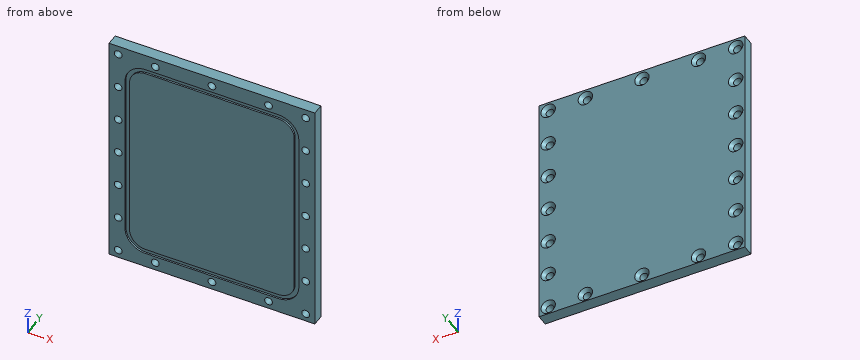
```python
from build123d import *

# Parameters (mm, degrees)
SKETCH1_W                                           = 90
SKETCH1_H                                           = 105
EXTRUDE1_DEPTH                                      = 5
CSK_FOR_M3_COUNTERSUNK_FLAT_HEAD_SCREW1_D           = 3.4
CSK_FOR_M3_COUNTERSUNK_FLAT_HEAD_SCREW1_CSINK_D     = 6.3
CSK_FOR_M3_COUNTERSUNK_FLAT_HEAD_SCREW1_CSINK_ANGLE = 90
EXTRUDE2_START                                      = -5
EXTRUDE2_DEPTH                                      = 0.75


with BuildPart() as part:
    # Sketch1 → Extrude1 (new body)
    with BuildSketch(Plane(origin=(0, 0, 0), x_dir=(1, 0, 0), z_dir=(0, 1, 0))):
        with Locations((45, 52.5)):
            Rectangle(SKETCH1_W, SKETCH1_H)
    extrude(amount=EXTRUDE1_DEPTH)

    # CSK for M3 Countersunk Flat Head Screw1 (through all)
    with Locations(Plane(origin=(4, 5, -4), x_dir=(0, 0, 1), z_dir=(0, 1, 0))):
        with Locations((0, 0), (-16.25, 0), (-32.5, 0), (-48.75, 0), (-65, 0), (-81.25, 0), (-97.5, 0), (-97.5, 16.25), (-97.5, 41), (-97.5, 65.75), (-97.5, 82), (-81.25, 82), (-65, 82), (-48.75, 82), (-32.5, 82), (-16.25, 82), (0, 82), (0, 65.75), (0, 41), (0, 16.25)):
            CounterSinkHole(CSK_FOR_M3_COUNTERSUNK_FLAT_HEAD_SCREW1_D / 2, CSK_FOR_M3_COUNTERSUNK_FLAT_HEAD_SCREW1_CSINK_D / 2, counter_sink_angle=CSK_FOR_M3_COUNTERSUNK_FLAT_HEAD_SCREW1_CSINK_ANGLE)

    # Sketch2 → Extrude2 (cut)
    with BuildSketch(Plane(origin=(0, 5, 0), x_dir=(1, 0, 0), z_dir=(0, 1, 0)).offset(EXTRUDE2_START)):
        with BuildLine():
            Line((16, 7), (74, 7))
            ThreePointArc((74, 7), (80.363961031, 9.636038969), (83, 16))
            Line((83, 16), (83, 89.5))
            ThreePointArc((83, 89.5), (80.363961031, 95.863961031), (74, 98.5))
            Line((74, 98.5), (16, 98.5))
            ThreePointArc((16, 98.5), (9.636038969, 95.863961031), (7, 89.5))
            Line((7, 89.5), (7, 16))
            ThreePointArc((7, 16), (9.636038969, 9.636038969), (16, 7))
        make_face()
        with BuildLine():
            Line((9, 89.5), (9, 16))
            ThreePointArc((9, 16), (11.050252532, 11.050252532), (16, 9))
            Line((16, 9), (74, 9))
            ThreePointArc((74, 9), (78.949747468, 11.050252532), (81, 16))
            Line((81, 16), (81, 89.5))
            ThreePointArc((81, 89.5), (78.949747468, 94.449747468), (74, 96.5))
            Line((74, 96.5), (16, 96.5))
            ThreePointArc((16, 96.5), (11.050252532, 94.449747468), (9, 89.5))
        make_face(mode=Mode.SUBTRACT)
    extrude(amount=EXTRUDE2_DEPTH, mode=Mode.SUBTRACT)


solid = part.part
```
Build history of the part. All positions in model axes, mm. Round coordinates to 2 decimals unless told otherwise and drop trailing zeros. Order: outer loops, then holes, each group sorted by start corner. A loop starts at its lowest first (then second) coordinate and runs counter-clockwise, first axis right, second up. Notation, with made-up numbers: (27.5, 52) -> (61.5, 52) arc R37 ccw to (61.5, 90) -> close; hole circle Ø8 at (35, -12). An arc over 180 degrees is marked (long way). Answer in a Markdown table with one row per item.
1) Band-saw the part on D-D on z = -69. Give the cut face in (x, y).
Values:
| item | result |
|---|---|
| outline | (0, 0) -> (2.3, 0) -> (2.3, 3.55) -> (0.85, 5) -> (0, 5) -> close; (5.7, 0) -> (7, 0) -> (7, 0.75) -> (9, 0.75) -> (9, 0) -> (81, 0) -> (81, 0.75) -> (83, 0.75) -> (83, 0) -> (84.3, 0) -> (84.3, 3.55) -> (82.85, 5) -> (7.15, 5) -> (5.7, 3.55) -> close; (87.7, 0) -> (90, 0) -> (90, 5) -> (89.15, 5) -> (87.7, 3.55) -> close |
2) Pin check, flat tips, straight feed: P1, Ø2, axis at x = 86, z = -20.25, coming from the -Y side; P2, Ø4, axis at x = 86, z = -4, coming from the +Y side; P3, Ø5.5, axis at x = 86, z = -52.75, coming from the +Y side. Stop position of each tip, or through.
Values:
| item | result |
|---|---|
| P1 | through |
| P2 | y = 3.85 |
| P3 | y = 4.6 |
3) Band-saw the part on B-B on x = 20.25. Give the cut face in (y, z), and give its area (3 significant figures).
Values:
| item | result |
|---|---|
| outline | (0, -105) -> (5, -105) -> (5, -104.65) -> (3.55, -103.2) -> (0, -103.2) -> close; (0, -99.8) -> (3.55, -99.8) -> (5, -98.35) -> (5, -7.15) -> (3.55, -5.7) -> (0, -5.7) -> (0, -7) -> (0.75, -7) -> (0.75, -9) -> (0, -9) -> (0, -96.5) -> (0.75, -96.5) -> (0.75, -98.5) -> (0, -98.5) -> close; (0, -2.3) -> (3.55, -2.3) -> (5, -0.85) -> (5, 0) -> (0, 0) -> close |
| area | 484 mm2 |
4) Band-saw the part on A-A on z = -4. Give the number of separate pieces and of enclosed holes in the cut face, and give its area (3 significant figures).
Values:
| item | result |
|---|---|
| separate pieces | 6 |
| enclosed holes | 0 |
| area | 354 mm2 |
5) Wall check: L1, parallel to Z at x = 69.75, y = 1.45; L2, parallel to X at y = 2, z = -101.5; L3, parallel to X at y = 3.2, z = -5.5. Give the ranges that are in metal, low to high.
Values:
| item | result |
|---|---|
| L1 | -105 to -103.2, -99.8 to -5.7, -2.3 to 0 |
| L2 | 0 to 2.3, 5.7 to 18.55, 21.95 to 43.3, 46.7 to 68.05, 71.45 to 84.3, 87.7 to 90 |
| L3 | 0 to 3.2, 4.8 to 19.45, 21.05 to 44.2, 45.8 to 68.95, 70.55 to 85.2, 86.8 to 90 |
